```python
from build123d import *

# Parameters (mm, degrees)
F1_DEPTH = 12.7
F2_W     = 2.54
F2_H     = 3.937
F3_DEPTH = 25.4
F4_R     = 1.524
F5_R     = 0.635
F6_DEPTH = 25.4


with BuildPart() as f1:
    # F0 (on Front) → F1 (new body)
    with BuildSketch(Plane.XZ):
        Polygon((-2.863529, 1.524), (-3.743411, 0), (3.622589, 0), (2.742708, 1.524), (5.488804, 1.524), (5.488804, 5.461), (-5.609625, 5.461), (-5.609625, 1.524), align=None)
    extrude(amount=F1_DEPTH)

    # F2 (on face) → F3 (intersect)
    with BuildSketch(Plane.YZ.offset(5.488804)):
        with Locations((-6.35, 3.4925)):
            Rectangle(F2_W, F2_H)
        Polygon((-7.62, 1.524), (-12.7, 1.524), (-12.7, 0), (0, 0), (0, 1.524), (-5.08, 1.524), align=None)
    extrude(amount=-F3_DEPTH, mode=Mode.INTERSECT)

    # F4
    f4_edges = [f1.edges().sort_by_distance(p)[0] for p in [
        (-5.609625, -6.35, 5.461),
    ]]
    fillet(f4_edges, radius=F4_R)

    # F5 (on face) → F6 (cut)
    with BuildSketch(Plane.YZ.offset(5.488804)):
        with Locations((-6.35, 4.445)):
            Circle(F5_R)
    extrude(amount=-F6_DEPTH, mode=Mode.SUBTRACT)


solid = f1.part
```
Design review of the part built by this model. Coordinates are the model's own, in mm. A direction names the side the tool comes from. Coordinates: 2 decimals unless noted, no trailing zeros. Order: outer loops, then holes, each group sorted by start corner. A loop starts at its lowest first (then second) coordinate and runs counter-clockwise, first axis right, second up.
1) Take a section at B-B, the plane x = 0. Give the boundary of the cut face in (y, z) (3 decimals).
2) Take a section at D-D, the plane y = -2.25. Give the boundary of the cut face in (x, z), and give its area (3 significant figures).
3) For faces 1 (the flat face through (-4, -6, 1.524)), 2 (the flat face through (0, -7.62, 3)), 3 (the flat face through (0, -5.08, 3)), list the 3-axis set-ups (+Z, -Z, +X, -X, +Y, -Y) from which the entire face can be reached by the end or side of a thin tool; tool diameter is ignored.
4) Clearance check with flat-ended pins moving along their axes: pin 1 (1.5 mm diameter, centred on x = -1.5, z = 4, fed in from +Y); pin 2 (2 mm diameter, centred on x = 1.5, y = -7.5, fed in from -Z); pin 3 (2 mm diameter, centred on x = 3.5, y = -10.5, fed in from +Z); pin 4 (3 mm diameter, centred on x = -2.5, z = 4.5, fed in from -Y). State where each tip first meets the part, or that it passes through.
5) Take a section at C-C, the plane y = -6.35. Give the boundary of the cut face in (x, z).
6) Wall thickness on line 1 along Z through (x, y) = (-2, -6.35); line 2 along Z through (x, y) = (3.25, -6.35); line 3 along Y through (x, z) = (-4.25, 5.2): over which ranges is each line inside the solid? List them lowest first.
7) Take a section at A-A, the plane z = 4.3. Give the boundary of the cut face in (x, y).
8) Mouldability with a two-part tool opening along Z and no side actions: class faces 4 (the flat face through (0, 0, 1)), 5 (the flat face through (4, -6, 1.524)), 6 (the flat face through (0, -10, 1.524)) as +Z half, -Z half, draft (parallel to the pull), parting line (faces both ways), or undercut.
Returned:
1. outline: (-12.7, 0) - (0, 0) - (0, 1.524) - (-5.08, 1.524) - (-5.08, 5.461) - (-7.62, 5.461) - (-7.62, 1.524) - (-12.7, 1.524) - close; hole circle Ø1.27 at (-6.35, 4.445)
2. outline: (-3.74, 0) - (3.62, 0) - (2.74, 1.52) - (-2.86, 1.52) - close
2. area: 9.88 mm2
3. face 1: -X, +Y, -Y
3. face 2: +Z, +X, -X, -Y
3. face 3: +Z, +X, -X, +Y
4. pin 1: stops at y = -5.08
4. pin 2: stops at z = 0
4. pin 3: stops at z = 1.52
4. pin 4: stops at y = -7.62
5. outline: (-5.61, 1.52) - (-2.86, 1.52) - (-3.74, 0) - (3.62, 0) - (2.74, 1.52) - (5.49, 1.52) - (5.49, 3.81) - (-5.61, 3.81) - close; (-5.09, 5.08) - (5.49, 5.08) - (5.49, 5.46) - (-4.09, 5.46) arc R1.52 ccw to start
6. line 1: z = 0 to 3.81, 5.08 to 5.46
6. line 2: z = 0 to 0.65, 1.52 to 3.81, 5.08 to 5.46
6. line 3: y = -7.62 to -5.08
7. outline: (-5.57, -7.62) - (5.49, -7.62) - (5.49, -6.97) - (-5.57, -6.97) - close; (-5.57, -5.73) - (5.49, -5.73) - (5.49, -5.08) - (-5.57, -5.08) - close
8. face 4: draft
8. face 5: undercut
8. face 6: +Z half
